```python
from build123d import *

# Parameters (mm, degrees)
F0_R     = 47.5
F1_DEPTH = 10
F2_R     = 5
F3_R     = 36.336935
F3_R_2   = 34.443129
F4_DEPTH = 2


with BuildPart() as f1:
    # F0 (on Top) → F1 (new body)
    with BuildSketch(Plane.XY):
        Circle(F0_R)
    extrude(amount=F1_DEPTH)

    # F2
    f2_edges = [f1.edges().sort_by_distance(p)[0] for p in [
        (-47.5, 0, 10),
    ]]
    fillet(f2_edges, radius=F2_R)

    # F3 (on face) → F4 (cut)
    with BuildSketch(Plane.XY.offset(10)):
        Circle(F3_R)
        Circle(F3_R_2, mode=Mode.SUBTRACT)
    extrude(amount=-F4_DEPTH, mode=Mode.SUBTRACT)


solid = f1.part
```
Check sheet for the modelled part. Datum: model origin and axes. Units: mm. A direction names the side the tool comes from. Round coordinates to 2 decimals unless told otherwise and drop trailing zeros. Loops run counter-clockwise (first coordinate to the right, second up) from the corner with the lowest first, then second, coordinate; pieces in that order, holes last. Notation, with made-up numbers: (40, 65) - (62, 65) arc R5 ccw to (62, 72) - close; hole circle Ø5 at (72.5, 71.25). An arc over 180 degrees is marked (long way). Write item = value, one per line. Start each with the question number.
Q1. Depth check by flat-ended pin: P1, Ø8, axis at x = 32.5, y = -37, coming from the -Z side; P2, Ø6, axis at y = 17, z = 5, coming from the -X side; P3, Ø2, axis at x = -12.5, z = 7.5, coming from the +Y side; P4, Ø3, axis at y = 14, z = 7, coming from the -X side. Enter the tip coordinate at first touch or a pass-through.
Q2. Thickness scan on L1, parallel to Y at x = 0, z = 8.9; L2, parallel to Y at x = -26, z = 9; L3, parallel to X at y = -6.5, z = 9. Record the ranges inside material, lowest first.
Q3. Release check for a two-part mould opening along Y. For faces 3 (the face through (-10.3, -46.37, 2.46)), 4 (the face through (31.3, 19.1, 10)), 5 (the face through (-7.877, -35.473, 9.014)) record: pulls with the +Y half, pulls with the -Y half, needs draft (parallel to the pull), parting line crosses it, or undercut.
Q4. Section check C-C (z = 2.5). Record the boundary of the cut face in (x, y), plus the area to 3 significant figures.
Q5. Access from +Z, -Z, +X, -X, +Y, -Y to the whole of each face (thin tool, end or side, straight path). Record for faces 1 (the face through (0, 0, 10)), 2 (the face through (-22, -27, 8)).
Q6. Section check A-A (y = 0). Record the boundary of the cut face in (x, z).
Derived:
q1.P1 = 0
q1.P2 = -45.39
q1.P3 = 45.68
q1.P4 = -45.62
q2.L1 = -45.63 to -36.34, -34.44 to 34.44, 36.34 to 45.63
q2.L2 = -37.34 to -25.38, -22.59 to 22.59, 25.38 to 37.34
q2.L3 = -45.03 to -35.75, -33.82 to 33.82, 35.75 to 45.03
q3.face_3 = parting line crosses it
q3.face_4 = needs draft
q3.face_5 = undercut
q4.outline = circle Ø95 at (0, 0)
q4.area = 7,090 mm^2
q5.face_1 = +Z, +X, -X, +Y, -Y
q5.face_2 = +Z
q6.outline = (-47.5, 0) - (47.5, 0) - (47.5, 5) arc R5 ccw to (42.5, 10) - (36.34, 10) - (36.34, 8) - (34.44, 8) - (34.44, 10) - (-34.44, 10) - (-34.44, 8) - (-36.34, 8) - (-36.34, 10) - (-42.5, 10) arc R5 ccw to (-47.5, 5) - close
